Design review of the part built by this model. Coordinates are the model's own, in mm. A direction names the side the tool comes from. Give positions to 0.01 mm unless a question says otherwise; leave off trailing zeros. Loops run counter-clockwise (first coordinate to the right, second up) from the corner with the lowest first, then second, coordinate; pieces in that order, holes last. Notation, with made-up numbers: M -5,13 L 34,13 A10 cw 34,18 Z; hole C 88.25,67 d10. An arc over 180 degrees is marked long. Use a Markdown table: item, result. Add a question column.
(1) Draft analysis for pull direction Y (two halves, no side actions). For faces 1 (the face through (0.69, -10.88, 1.21)), 2 (the face through (-5.71, 1.4, 0.9)), 3 (the face through (1, 4, 0)), state which applies: pulls with the +Y half, pulls with the -Y half, needs draft (parallel to the pull), parting line crosses it, or undercut.
(2) For faces 4 (the face through (-41.062, 1.322, 0.781)), 5 (the face through (5.715, -7.771, 0.702)), 6 (the face through (-28.61, -3.21, 0.78)), list the 3-axis set-ups (+Z, -Z, +X, -X, +Y, -Y) from which the entire face can be reached by the end or side of a thin tool; tool diameter is ignored.
(3) Add section A-A, the plane x = -1. Give the boundary of the cut face in (y, z), then the cut area to 3 significant figures.
(4) Add section B-B, the plane z = 1.35. State how many separate pieces and enclosed holes the cut face has, then the cut area to 3 significant figures.
(5) Add section C-C, the plane x = 20.5. Give the boundary of the cut face in (y, z), then the cut area to 3 significant figures.
(6) For probe 1 along X at (y, z) = (-3, 1.3); probe 2 along Y at (x, z) = (-31, 0.25); probe 3 along Y at (x, z) = (14, 0.8), list the stretches that pass through material, from the lowest coordinate up.
(7) Add section D-D, the plane x = -33. Give the boundary of the cut face in (y, z), then the cut area to 3 significant figures.
```python
from build123d import *

# Parameters (mm, degrees)
CROQUIS1_W              = 98
CROQUIS1_H              = 20
SALIENTE_EXTRUIR1_DEPTH = 1.6
SALIENTE_EXTRUIR2_DEPTH = 98
CORTAR_EXTRUIR1_START   = -8
CORTAR_EXTRUIR1_DEPTH   = 20
CORTAR_EXTRUIR2_REACH   = 91.04


with BuildPart() as part:
    # Croquis1 → Saliente-Extruir1 (new body)
    with BuildSketch(Plane.XY):
        Rectangle(CROQUIS1_W, CROQUIS1_H)
    extrude(amount=SALIENTE_EXTRUIR1_DEPTH)

    # Croquis2 → Saliente-Extruir2 (add)
    with BuildSketch(Plane(origin=(49, 0, 0), x_dir=(0, 0, -1), z_dir=(1, 0, 0))):
        Polygon((0, -11.359205127), (-0.837384271, -11.728681668), (-1.6, -10), (0, -10), align=None)
    extrude(amount=-SALIENTE_EXTRUIR2_DEPTH)

    # Croquis3 → Cortar-Extruir1 (cut)
    with BuildSketch(Plane(origin=(0, -10.293644781, -14.534478238), x_dir=(-1, 0, 0), z_dir=(0, 0.42110532053516664, -0.9070117469013147)).offset(CORTAR_EXTRUIR1_START)):
        with BuildLine():
            Line((6, 9.403690819), (6, 16.403690819))
            ThreePointArc((6, 16.403690819), (5.707106781, 17.1107976), (5, 17.403690819))
            Line((5, 17.403690819), (-5, 17.403690819))
            ThreePointArc((-5, 17.403690819), (-5.707106781, 17.1107976), (-6, 16.403690819))
            Line((-6, 16.403690819), (-6, 9.403690819))
            ThreePointArc((-6, 9.403690819), (-5.707106781, 8.696584037), (-5, 8.403690819))
            Line((-5, 8.403690819), (5, 8.403690819))
            ThreePointArc((5, 8.403690819), (5.707106781, 8.696584037), (6, 9.403690819))
        make_face()
    extrude(amount=-CORTAR_EXTRUIR1_DEPTH, mode=Mode.SUBTRACT)

    # Cortar-Extruir2: from a plane face, 91.04 long prism both ways, kept between that surface and its translate by the depth
    cortar_extruir2_start = Plane(origin=(0, 0, 1.6), z_dir=(0, 0, -1)) * Box(366.16, 366.16, 183.08, align=(Align.CENTER, Align.CENTER, Align.MIN), mode=Mode.PRIVATE)
    cortar_extruir2_end = Plane(origin=(-9.998158796, 7.340799912, -14.089151581), z_dir=(0, 0, -1)) * Box(366.16, 366.16, 183.08, align=(Align.CENTER, Align.CENTER, Align.MIN), mode=Mode.PRIVATE)
    # Croquis4 → Cortar-Extruir2 (cut, from a surface)
    with BuildSketch(Plane(origin=(15.242771226, -12.659892112, -9.623968273), x_dir=(-0.8660785482382583, -0.21185862229734287, 0.4527956188389888), z_dir=(-0.49990793980643183, 0.36703999560816625, -0.7844575790585788)), mode=Mode.PRIVATE) as cortar_extruir2_sk1:
        with BuildLine():
            Line((-8.828097078, 9.489452405), (-8.905642597, 16.48902287))
            ThreePointArc((-8.905642597, 16.48902287), (-9.206351123, 17.19284161), (-9.916659166, 17.477883576))
            Line((-9.916659166, 17.477883576), (-19.916045544, 17.367104263))
            ThreePointArc((-19.916045544, 17.367104263), (-20.619864285, 17.066395736), (-20.904906251, 16.356087694))
            Line((-20.904906251, 16.356087694), (-20.827360732, 9.356517229))
            ThreePointArc((-20.827360732, 9.356517229), (-20.526652205, 8.652698488), (-19.816344162, 8.367656522))
            Line((-19.816344162, 8.367656522), (-9.816957784, 8.478435835))
            ThreePointArc((-9.816957784, 8.478435835), (-9.113139043, 8.779144362), (-8.828097078, 9.489452405))
        make_face()
    cortar_extruir2_tool1 = extrude(cortar_extruir2_sk1.sketch, amount=CORTAR_EXTRUIR2_REACH, both=True, mode=Mode.PRIVATE)
    cortar_extruir2 = ((cortar_extruir2_tool1 & cortar_extruir2_start) - cortar_extruir2_end).solids().sort_by_distance((35.560858, -3.26981, 0.8))[0]
    add(cortar_extruir2, mode=Mode.SUBTRACT)

    # Simetría1: Cortar-Extruir2 across plane
    add(cortar_extruir2.mirror(Plane(origin=(0, 0, 0), x_dir=(0, 0, 1), z_dir=(1, 0, 0))), mode=Mode.SUBTRACT)


solid = part.part
```
Established:
| question | item | result |
|---|---|---|
| 1 | face 1 | pulls with the -Y half |
| 1 | face 2 | undercut |
| 1 | face 3 | needs draft |
| 2 | face 4 | none |
| 2 | face 5 | +Z |
| 2 | face 6 | -Z |
| 3 | outline | M -11.73,0.84 L -11.36,0 L -7.78,0 L -8.52,1.6 L -10,1.6 Z; M 1.4,1.6 L 2.12,0.05 L 2.01,0 L 10,0 L 10,1.6 Z |
| 3 | area | 18.1 mm^2 |
| 4 | separate pieces | 1 |
| 4 | enclosed holes | 3 |
| 4 | area | 1,620 mm^2 |
| 5 | outline | M -11.73,0.84 L -11.36,0 L 10,0 L 10,1.6 L -10,1.6 Z |
| 5 | area | 34.0 mm^2 |
| 6 | probe 1 | -49 to -42.69, -28.83 to -6, 6 to 28.83, 42.69 to 49 |
| 6 | probe 2 | -11.47 to -7.92, 1.99 to 10 |
| 6 | probe 3 | -11.71 to 10 |
| 7 | outline | M -11.73,0.84 L -11.36,0 L -7.83,0 L -8.57,1.6 L -10,1.6 Z; M 1.34,1.6 L 2.08,0 L 10,0 L 10,1.6 Z |
| 7 | area | 18.1 mm^2 |
